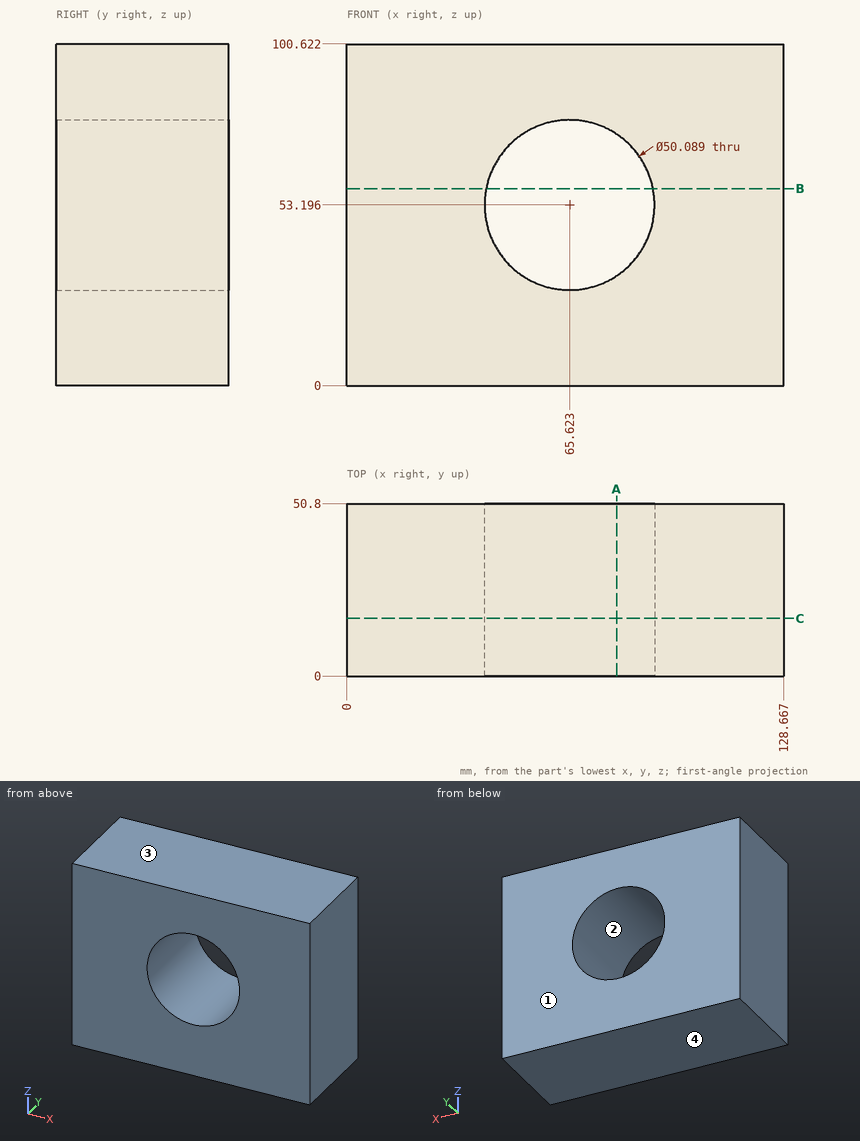
The figure shows three views and two pictorial views of one solid part (mm, origin at its lowest corner). Answer the questions. Round coordinates to 2 decimals unless told otherwise and drop trailing zeros. Loops run counter-clockwise (first coordinate to the right, second up) from the corner with the lowest first, then second, coordinate; pieces in that order, holes last. Notation, with made-up numbers: (-30, 48.5) - (-14, 48.5) arc R16 ccw to (-14, 63.5) - close; hole circle Ø2 at (11, 70.5). An arc over 180 degrees is marked (long way). Use one line per item in the form item = value. Start each with the question number.
(1) Consider line 1 (Z direction, x = 52, y = 41); line 2 (Z direction, x = 77, y = 35.5) (1 decimal); line 3 (X direction, y = 5, z = 71) (1 decimal). Determine where each line is inside the solid, lowest interval first.
(2) Find section C-C on y = 17. Determine the outline of the cut face in (x, z) (1 decimal), and give its area (3 significant figures).
(3) Find section A-A on x = 79.5. Determine the outline of the cut face in (y, z).
(4) Find section B-B on z = 58. Determine the outline of the cut face in (x, y), and give its area (3 significant figures).
(5) Determine the mould class of the marked faces 1, 2, 3 and 4 for opening direction Z: +Z half, -Z half, draft (parallel to the pull), parting line (faces both ways), or undercut.
Answer list:
q1.line_1 = 0 to 32.18, 74.21 to 100.62
q1.line_2 = 0 to 30.9, 75.5 to 100.6
q1.line_3 = 0 to 48, 83.2 to 128.7
q2.outline = (0, 0) - (128.7, 0) - (128.7, 100.6) - (0, 100.6) - close; hole circle Ø50.1 at (65.6, 53.2)
q2.area = 11,000 mm^2
q3.outline = (0, 0) - (50.8, 0) - (50.8, 32.35) - (0, 32.35) - close; (0, 74.04) - (50.8, 74.04) - (50.8, 100.62) - (0, 100.62) - close
q4.outline = (0, 0) - (41.04, 0) - (41.04, 50.8) - (0, 50.8) - close; (90.2, 0) - (128.67, 0) - (128.67, 50.8) - (90.2, 50.8) - close
q4.area = 4,040 mm^2
q5.face_1 = draft
q5.face_2 = undercut
q5.face_3 = +Z half
q5.face_4 = -Z half
